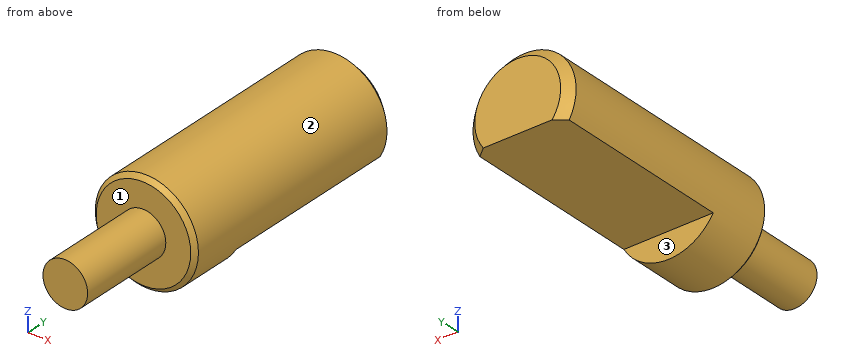
```python
from build123d import *

# Parameters (mm, degrees)
SKETCH_1_R          = 1.3
EXTRUDE_1_DEPTH     = 5.7
SKETCH_2_R          = 3
EXTRUDE_2_DEPTH     = 14.5
CHAMFER_1_SIZE      = 0.25
CUT_EXTRUDE_1_DEPTH = 11
CHAMFER_2_SIZE      = 0.5


with BuildPart() as part:
    # 草图1 → 凸台-拉伸1 (new body)
    with BuildSketch(Plane(origin=(0, 0, 0), x_dir=(1, 0, 0), z_dir=(0, 1, 0))):
        Circle(SKETCH_1_R)
    extrude(amount=EXTRUDE_1_DEPTH)

    # 草图2 → 凸台-拉伸2 (add)
    with BuildSketch(Plane(origin=(0, 5.7, 0), x_dir=(1, 0, 0), z_dir=(0, 1, 0))):
        Circle(SKETCH_2_R)
    extrude(amount=EXTRUDE_2_DEPTH)

    # 倒角1
    chamfer_1_edges = [part.edges().sort_by_distance(p)[0] for p in [
        (-3, 5.7, 0),
    ]]
    chamfer(chamfer_1_edges, length=CHAMFER_1_SIZE)

    # 草图3 → 切除-拉伸1 (cut)
    with BuildSketch(Plane(origin=(0, 20.2, 0), x_dir=(1, 0, 0), z_dir=(0, 1, 0))):
        with BuildLine():
            Line((-2.598076211, 1.5), (2.598076211, 1.5))
            ThreePointArc((2.598076211, 1.5), (0, 3), (-2.598076211, 1.5))
        make_face()
    extrude(amount=-CUT_EXTRUDE_1_DEPTH, mode=Mode.SUBTRACT)

    # 倒角2
    chamfer_2_edges = [part.edges().sort_by_distance(p)[0] for p in [
        (-0.776457135, 20.2, 2.897777479),
    ]]
    chamfer(chamfer_2_edges, length=CHAMFER_2_SIZE)


solid = part.part
```
Geometry check sheet. Reference: the model listing, model coordinates, mm. Face numbers are marked on the shaded views. A direction names the side the tool comes from. Give positions to 0.01 mm unless a question says otherwise; leave off trailing zeros. Order: outer loops, then holes, each group sorted by start corner. A loop starts at its lowest first (then second) coordinate and runs counter-clockwise, first axis right, second up. Notation, with made-up numbers: (-11, 23) -> (4, 23) arc R23 cw to (4, 48) -> close; hole circle Ø4 at (1, 88). An arc over 180 degrees is marked (long way). Write each question's results on one line, items separated by ' | '. Start each with the question number.
(1) Gauge pin test, flat ends, axial feed: P1, Ø1, axis at y = 16.5, z = 1, coming from the -X side; P2, Ø0.8, axis at x = -0.5, z = -2.5, coming from the +Y side. Record the tip position at first contact, or that the pin passes through.
(2) Sectioned sample at C-C (y = 2.25). Enter the section's corners in (x, z), plus the area to 3 significant figures.
(3) Sectioned sample at A-A (z = 0). Enter the section's corners in (x, y).
(4) Sectioned sample at D-D (y = 10.5). Enter the section's corners in (x, z), plus the area to 3 significant figures.
(5) Scan lines: line 1 (Y direction, x = 1.1, z = -2.25); line 2 (Y direction, x = -0.2, z = 1.45); line 3 (Z direction, x = 0.05, y = 15). Record each from-to range of solid material in increasing order.
(6) Access from +Z, -Z, +X, -X, +Y, -Y to the whole of each face (thin tool, end or side, straight path). Record for the marked faces 1, 2 and 3.
(7) Sectioned sample at B-B (x = 0). Enter the section's corners in (y, z), plus the area to 3 significant figures.
Answer below:
1) P1: x = -2.96 | P2: y = 9.2
2) outline: circle Ø2.6 at (0, 0) | area: 5.31 mm2
3) outline: (-3, 5.95) -> (-2.75, 5.7) -> (-1.3, 5.7) -> (-1.3, 0) -> (1.3, 0) -> (1.3, 5.7) -> (2.75, 5.7) -> (3, 5.95) -> (3, 19.7) -> (2.5, 20.2) -> (-2.5, 20.2) -> (-3, 19.7) -> close
4) outline: (-2.6, -1.5) -> (2.6, -1.5) arc R3 ccw (long way) to start | area: 22.7 mm2
5) line 1: 5.7 to 9.2 | line 2: 5.7 to 20.2 | line 3: -1.5 to 3
6) face 1: -Y | face 2: +Y, -Y | face 3: -Z, +X, -X, +Y
7) outline: (0, -1.3) -> (5.7, -1.3) -> (5.7, -2.75) -> (5.95, -3) -> (9.2, -3) -> (9.2, -1.5) -> (20.2, -1.5) -> (20.2, 2.5) -> (19.7, 3) -> (5.95, 3) -> (5.7, 2.75) -> (5.7, 1.3) -> (0, 1.3) -> close | area: 85.1 mm2
